Check sheet for the modelled part. Datum: model origin and axes. Units: mm. A direction names the side the tool comes from. Give positions to 0.01 mm unless a question says otherwise; leave off trailing zeros. Loops run counter-clockwise (first coordinate to the right, second up) from the corner with the lowest first, then second, coordinate; pieces in that order, holes last. Notation, with made-up numbers: M -18.5,74.5 L -5.5,74.5 A9 ccw -5.5,78.5 Z; hole C 25,-29 d2. An arc over 180 degrees is marked long. Write each question's results on one line, items separated by ' | '. Start each with the question number.
1. Draft check along Y on faces 3 (the flat face through (-1, 0, 24)), 4 (the cylindrical face through (-0.07, 1.48, 59.18)), 5 (the cylindrical face through (-0.3, 5.984, -13.933)). Enter one of: pulls with the +Y half, pulls with the -Y half, needs draft (parallel to the pull), parting line crosses it, or undercut.
2. Sectioned sample at B-B on x = -3. Record the cut outline in (y, z).
3. Tool access check on faces 1 (the flat face through (-1, 3, 26)), 2 (the flat face through (-1, 15, -14)). Record the directions out of +Z, -Z, +X, -X, +Y, -Y that give a thin tool (end or side, any length) a straight path to the whole face; none if there is none.
4. Sectioned sample at C-C on x = 3.25. Record the cut outline in (y, z), and give its area (3 significant figures).
5. Material ranges on line 1 along X through (y, z) = (11, -13.4); line 2 along Z through (x, y) = (-0.75, 5); line 3 along Y through (x, z) = (1.25, -5), recorded low to high.
6. Sectioned sample at A-A on y = 7. Record the cut outline in (x, z), and give its area (3 significant figures).
7. Go/stop test with flat-tipped pins: pin 1 (5 mm diameter, centred on x = 1, y = 8, fed in from +Z); pin 2 (1.3 mm diameter, centred on x = -0.72, y = 11, fed in from +Z); pin 3 (1 mm diameter, centred on x = -4, z = 10.5, fed in from -Y); pin 4 (2 mm diameter, centred on x = 0, z = 17, fed in from +Y). Record where each tip stops, or that it passes through.
8. Sectioned sample at D-D on z = 52.5. Record the cut outline in (x, y).
Autodesk Inventor part; units mm, degrees
ref_plane "YZ Plane" through (0, 0, 0) normal (1, 0, 0) x (0, 1, 0)
ref_plane "XZ Plane" through (0, 0, 0) normal (0, 1, 0) x (-1, 0, 0)
ref_plane "XY Plane" through (0, 0, 0) normal (0, 0, 1) x (1, 0, 0)
sketch "Sketch1" plane through (0, 0, 0) normal (0, 1, 0) x (-1, 0, 0)
  line L0 (-4.2784, 62.5876) -> (5.7216, 62.5876)
  line L1 (5.7216, 62.5876) -> (5.7216, -15.4124)
  line L2 (5.7216, -15.4124) -> (-4.2784, -15.4124)
  line L3 (-4.2784, -15.4124) -> (-4.2784, 62.5876)
  line L4 (-4.2784, -15.4124) -> (5.7216, -15.4124)
  line L5 (5.7216, -15.4124) -> (5.7216, -12.4124)
  line L6 (5.7216, -12.4124) -> (-4.2784, -12.4124)
  line L7 (-4.2784, -12.4124) -> (-4.2784, -15.4124)
  circle A0 centre (0.7216, 56.2526) radius 3
  point P0 (0, 0)
  dimension "d0" = 10
  dimension "d1" = 78
  dimension "d2" = 6.335
  dimension "d3" = 3
  dimension "d16" = 6
extrude "Extrusion1" add sketch "Sketch1" along normal blind 3 contours L0 L1 L6 L3
extrude "Extrusion2" add sketch "Sketch1" along normal blind 15 contours L6 L1 L2 L3
sketch "Sketch2" plane through (-5.7216, 3, -12.4124) normal (0, 0, 1) x (1, 0, 0)
  line L0 (0, 0) -> (0, 12)
  line L1 (0, 0) -> (10, 0)
  line L2 (5, 4) -> (5, 8) construction
  point P0 (5.7216, -3)
  point P1 (5, 0)
  point P2 (0, 6)
  point P3 (5, 6)
  dimension "d8" = 4
hole "Hole1" at (-0.7216, 11, -12.4124) at (-0.7216, 7, -12.4124) direction (0, 0, -1) diameter 2.2 end through all
properties part number "ALPHA_001158_Electrode8-mountbracket"
Output values:
1) face 3: pulls with the -Y half | face 4: needs draft | face 5: undercut
2) outline: M 0,-15.41 L 15,-15.41 L 15,-12.41 L 3,-12.41 L 3,54.3 L 0,54.3 Z; M 0,58.2 L 3,58.2 L 3,62.59 L 0,62.59 Z
3) face 1: +Z, +X, -X, +Y | face 2: +Z, -Z, +X, -X, +Y
4) outline: M 0,-15.41 L 15,-15.41 L 15,-12.41 L 3,-12.41 L 3,62.59 L 0,62.59 Z | area: 270 mm2
5) line 1: -5.72 to -1.82, 0.38 to 4.28 | line 2: -15.41 to -12.41 | line 3: 0 to 3
6) outline: M -5.72,-15.41 L -1.82,-15.41 L -1.82,-12.41 L -5.72,-12.41 Z; M 0.38,-15.41 L 4.28,-15.41 L 4.28,-12.41 L 0.38,-12.41 Z | area: 23.4 mm2
7) pin 1: z = -12.41 | pin 2: through | pin 3: y = 0 | pin 4: y = 3
8) outline: M -5.72,0 L 4.28,0 L 4.28,3 L -5.72,3 Z
